```python
from build123d import *

# Parameters (mm, degrees)
SKETCH_1_W      = 12.4
SKETCH_1_H      = 5
EXTRUDE_1_DEPTH = 2.54
SKETCH_2_R      = 0.4
EXTRUDE_2_DEPTH = 5.08


with BuildPart() as part:
    # 草图1 → 凸台-拉伸1 (new body)
    with BuildSketch(Plane.XY):
        with Locations((6.2, -2.5)):
            Rectangle(SKETCH_1_W, SKETCH_1_H)
    extrude(amount=EXTRUDE_1_DEPTH)

    # 草图2 → 凸台-拉伸2 (add, symmetric)
    with BuildSketch(Plane.XY.offset(2.54)):
        with Locations((6.2, -1.23)):
            Circle(SKETCH_2_R)
        with Locations((8.74, -1.23)):
            Circle(SKETCH_2_R)
        with Locations((11.28, -1.23)):
            Circle(SKETCH_2_R)
        with Locations(Location((1.12, -1.23, 0), (0, 0, 180))):
            Circle(SKETCH_2_R)
        with Locations(Location((3.66, -1.23, 0), (0, 0, 180))):
            Circle(SKETCH_2_R)
        with Locations(Location((11.28, -3.77, 0), (0, 0, 180))):
            Circle(SKETCH_2_R)
        with Locations(Location((8.74, -3.77, 0), (0, 0, 180))):
            Circle(SKETCH_2_R)
        with Locations(Location((6.2, -3.77, 0), (0, 0, 180))):
            Circle(SKETCH_2_R)
        with Locations((3.66, -3.77)):
            Circle(SKETCH_2_R)
        with Locations((1.12, -3.77)):
            Circle(SKETCH_2_R)
    extrude(amount=EXTRUDE_2_DEPTH, both=True)


solid = part.part
```
Read the model definition and answer for the solid it produces. Units are mm, in the model's axes. A direction names the side the tool comes from. Coordinates: 2 decimals unless noted, no trailing zeros. Order: outer loops, then holes, each group sorted by start corner. A loop starts at its lowest first (then second) coordinate and runs counter-clockwise, first axis right, second up. Notation, with made-up numbers: (-35, -31) - (8, -31) arc R16 cw to (8, -22) - close; hole circle Ø5 at (-23.75, 45.5). An arc over 180 degrees is marked (long way). Answer as a JSON object with one key per item and string values. Group by question number.
Item 1: Section C-C (y = -4.5) is taken. Give the vertices of the cut face in (x, z).
Item 2: Consider probe 1 along Z at (x, y) = (3.25, -1.6); probe 2 along X at (y, z) = (-3.5, 5.25); probe 3 along Y at (x, z) = (8.5, 6.5). Determine where each line is inside the solid, lowest interval first. Write a range as from..to.
Item 3: A flat-ended cylindrical pin translates along its axis: P1, Ø1.5, axis at x = 4, y = -2.5, coming from the +Z side. Find the tip coordinate at first contact, or state that the pin passes through.
Item 4: Section A-A (z = -0.25) is taken. State how many separate pieces and enclosed holes the cut face has, plus the area to 3 significant figures.
Item 5: A tool of negligible diameter and unlimited length cuts with its end or side. For faces 4 (the face through (3.29, -1.08, 5.04)), 5 (the face through (11.095, -3.415, -1.252)), from which of +Z, -Z, +X, -X, +Y, -Y can it reach the whole face along a straight path? Write none if from no direction.
Item 6: The mould has two halves that part along Y. Classify faces 1 (the face through (6, 0, 1)), 2 (the face through (10.985, -0.96, 5.044)), 3 (the face through (0, -3, 1)): +Y half, -Y half, draft (parallel to the pull), parting line (faces both ways), or undercut.
Item 7: Section B-B (x = 8.74) is taken. Give the vertices of the cut face in (y, z).
Results are:
{
 "1": {"outline": "(0, 0) - (12.4, 0) - (12.4, 2.54) - (0, 2.54) - close"},
 "2": {"probe 1": "z = 0..2.54", "probe 2": "x = 0.82..1.42, 3.36..3.96, 5.9..6.5, 8.44..9.04, 10.98..11.58", "probe 3": "y = -4.09..-3.45, -1.55..-0.91"},
 "3": {"P1": "stops at z = 2.54"},
 "4": {"separate pieces": "10", "enclosed holes": "0", "area": "5.03 mm^2"},
 "5": {"face 4": "+Z", "face 5": "-Z"},
 "6": {"face 1": "+Y half", "face 2": "undercut", "face 3": "draft"},
 "7": {"outline": "(-5, 0) - (-4.17, 0) - (-4.17, -2.54) - (-3.37, -2.54) - (-3.37, 0) - (-1.63, 0) - (-1.63, -2.54) - (-0.83, -2.54) - (-0.83, 0) - (0, 0) - (0, 2.54) - (-0.83, 2.54) - (-0.83, 7.62) - (-1.63, 7.62) - (-1.63, 2.54) - (-3.37, 2.54) - (-3.37, 7.62) - (-4.17, 7.62) - (-4.17, 2.54) - (-5, 2.54) - close"}
}
